from build123d import *

# Parameters (mm, degrees)
F1_DEPTH = 6.35
F3_DEPTH = 12.701
F6_R     = 2.54
F7_SIZE  = 2.54
F8_R     = 2.54


with BuildPart() as f1:
    # F0 (on Top) → F1 (new body, symmetric)
    with BuildSketch(Plane.XY):
        with BuildLine():
            Line((21.59, 7.62), (-21.59, 7.62))
            ThreePointArc((-21.59, 7.62), (-44.45, 0), (-21.59, -7.62))
            Line((-21.59, -7.62), (21.59, -7.62))
            ThreePointArc((21.59, -7.62), (44.45, 0), (21.59, 7.62))
        make_face()
    extrude(amount=F1_DEPTH, both=True)

    # F4: F3 across plane


with BuildPart() as f3:
    # F2 (on face) → F3 (new body, through all)
    with BuildSketch(Plane.XY.offset(6.35)):
        Polygon((-27.8347122138, 0), (-32.9673561069, 8.89), (-43.2326438931, 8.89), (-48.3652877862, 0), (-43.2326438931, -8.89), (-32.9673561069, -8.89), align=None)
    extrude(amount=-F3_DEPTH)


with BuildPart() as f1_1:
    add(f1.part)
    add(f3.part.mirror(Plane.YZ), mode=Mode.SUBTRACT)

    # F5: cut F3
    add(f3.part, mode=Mode.SUBTRACT)

    # F6
    f6_edges = [f1_1.edges().sort_by_distance(p)[0] for p in [
        (0, -7.62, 6.35),
        (-30.913065, -12.672393, 6.35),
        (-30.913065, 12.672393, 6.35),
        (0, 7.62, 6.35),
        (30.913065, 12.672393, 6.35),
        (30.913065, -12.672393, 6.35),
    ]]
    fillet(f6_edges, radius=F6_R)

    # F7
    f7_edges = [f1_1.edges().sort_by_distance(p)[0] for p in [
        (-30.913065, -12.672393, -6.35),
        (0, -7.62, -6.35),
        (30.913065, -12.672393, -6.35),
        (30.913065, 12.672393, -6.35),
        (0, 7.62, -6.35),
        (-30.913065, 12.672393, -6.35),
    ]]
    chamfer(f7_edges, length=F7_SIZE)

    # F8
    f8_edges = [f1_1.edges().sort_by_distance(p)[0] for p in [
        (-29.031016, -9.789419, -6.35),
        (0, -5.08, -6.35),
        (29.031016, -9.789419, -6.35),
        (29.031016, 9.789419, -6.35),
        (0, 5.08, -6.35),
        (-29.031016, 9.789419, -6.35),
    ]]
    fillet(f8_edges, radius=F8_R)


solid = f1_1.part
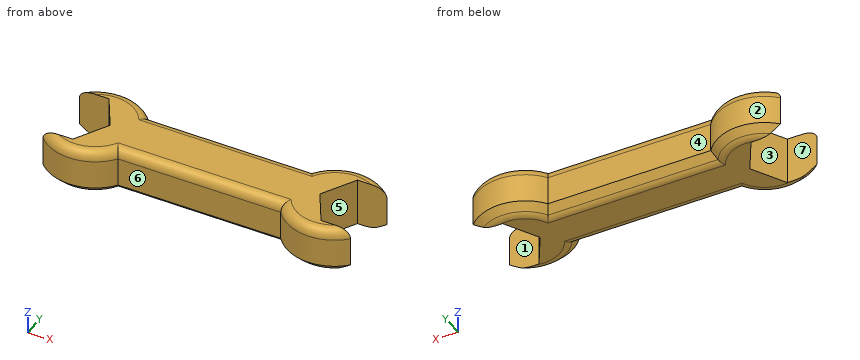
Geometry: final body of the model. Coordinates: model frame, mm. Face numbers are marked on the shaded views. A direction names the side the tool comes from. Round coordinates to 2 decimals unless told otherwise and drop trailing zeros. Loops run counter-clockwise (first coordinate to the right, second up) from the corner with the lowest first, then second, coordinate; pieces in that order, holes last. Notation, with made-up numbers: M -12,-13.5 L 47,-13.5 A22 ccw 47,3.5 Z; hole C 62,-15.75 d8. An arc over 180 degrees is marked long. One line per question, with ' | ' between items.
(1) Material intervals for line 1 along Y through (x, z) = (-31.5, 0.75); line 2 along Y through (x, z) = (10, -1); line 3 along X through (y, z) = (-9.5, 5), sorted ascending. Write a range as from..to.
Check result:
line 1: y = -12.7..-6.35, 6.35..12.7 | line 2: y = -7.62..7.62 | line 3: x = -39.73..-23.77, 23.77..39.73
(2) Cut plane A-A on z = -2.5. Return the cut outline in (x, y), plus the area to 3 significant figures.
Check result:
outline: M -40.82,-8.89 A12.7 ccw -21.59,-7.62 L 21.59,-7.62 A12.7 ccw 40.82,-8.89 L 32.97,-8.89 L 27.83,0 L 32.97,8.89 L 40.82,8.89 A12.7 ccw 21.59,7.62 L -21.59,7.62 A12.7 ccw -40.82,8.89 L -32.97,8.89 L -27.83,0 L -32.97,-8.89 Z | area: 1,160 mm2
(3) Cut plane B-B on x = -20.5. Return the cut outline in (y, z).
Check result:
outline: M -7.62,-3.81 L -5.82,-5.61 A2.54 ccw -4.03,-6.35 L 4.03,-6.35 A2.54 ccw 5.82,-5.61 L 7.62,-3.81 L 7.62,3.81 A2.54 ccw 5.08,6.35 L -5.08,6.35 A2.54 ccw -7.62,3.81 Z
(4) Access query for the marked faces 4, 5, 6 and 7. Directions: +Z, -Z, +X, -X, +Y, -Y. A direction counts if a zero-diameter tool reaches every point of the face in a straight line with its end or side. Return the directions, or none.
Check result:
face 4: +Z, -Z, +Y | face 5: +Z, -Z, +X | face 6: +Z, -Z, -Y | face 7: +Z, -Z, -X
(5) Pull-direction query (X, two-part tool) for the marked faces 1, 2 and 3; classes: +X half, -X half, draft (parallel to the pull), parting line (faces both ways), or undercut.
Check result:
face 1: draft | face 2: undercut | face 3: -X half
(6) Contact query for flat-ended pins moving along their axis: P1, Ø6.5, axis at x = -36, z = 0, coming from the +Y side; P2, Ø4, axis at x = -38, z = 0, coming from the -Y side; P3, Ø2.5, axis at x = 2, z = -1, coming from the +Y side. Output: stop coordinate, or through.
Check result:
P1: stops at y = 12.66 | P2: stops at y = -11.97 | P3: stops at y = 7.62
